For this review, take the finished solid that the model builds, in its own axes (mm). A direction names the side the tool comes from. Coordinates: 2 decimals unless noted, no trailing zeros. Write each loop counter-clockwise with the first axis right and the second up, starting at its lowest first coordinate (ties: lowest second). Pieces come first, ordered by that corner, then holes. Notation, with made-up numbers: (31, -36.75) -> (88, -36.75) arc R23 ccw to (88, -20.75) -> close; hole circle Ø7 at (6.25, -36). An arc over 180 degrees is marked (long way). One line per item, written item: value. Start each with the question number.
1) Add section A-A (z = -6.5). State the section outline as (x, y) points, and give its area (3 significant figures).
2) For probe 1 along X at (y, z) = (13, -11.5); probe 2 along Z at (x, y) = (27.5, -68.5); probe 3 along Y at (x, z) = (-10, -6.5), list the stretches that pass through material, from the lowest coordinate up. Write a range as from..to.
3) Machinability: for faces 4 (the flat face through (11, 70, -7)), 5 (the flat face through (11, -70, -7)), 6 (the flat face through (-7, -1, -7)), 7 (the flat face through (-15, -1, -7)), 8 (the flat face through (15, -1, -7)), which of the approach directions +Z, -Z, +X, -X, +Y, -Y give a long, thin tool a straight path to every point of the face, cutting with its end or side? Answer none if there is none.
4) Mouldability with a two-part tool opening along X and no side actions: class faces 1 (the flat face through (7, -1, -7)), 2 (the flat face through (-1, -90, 2)), 3 (the flat face through (-60, -3, 2)) as released by +X, released by -X, zero draft, split by the parting line, or undercut.
5) Add section B-B (y = -6.5). State the section outline as (x, z) points, and give its area (3 significant figures).
6) For pin 1 Ø8 at (x, y) = (22, 8.5) entering from -Z; pin 2 Ø1.5 at (y, z) = (-28.5, -11) entering from +X; pin 3 Ø4 at (x, z) = (-12.5, -9) entering from +Y, all flat-tipped, find the tip position at first contact; note any pin that passes through.
7) Add section C-C (x = -1.5). State the section outline as (y, z) points, and give its area (4 significant figures).
8) Add section D-D (y = -76). State the section outline as (x, z) points, and give its area (3 significant figures).
from build123d import *

# Parameters (mm, degrees)
SKETCH1_W           = 120
SKETCH1_H           = 180
BOSS_EXTRUDE1_DEPTH = 5
SKETCH2_W           = 8
SKETCH2_H           = 140
BOSS_EXTRUDE2_DEPTH = 14
SKETCH3_W           = 120
SKETCH3_H           = 3.5
CUT_EXTRUDE1_DEPTH  = 10


with BuildPart() as part:
    # Sketch1 → Boss-Extrude1 (new body)
    with BuildSketch(Plane.XY):
        Rectangle(SKETCH1_W, SKETCH1_H)
    extrude(amount=BOSS_EXTRUDE1_DEPTH)

    # Sketch2 → Boss-Extrude2 (add)
    with BuildSketch(Plane(origin=(0, 0, 0), x_dir=(-1, 0, 0), z_dir=(0, 0, -1))):
        with Locations((-11, 0)):
            Rectangle(SKETCH2_W, SKETCH2_H)
        with Locations((11, 0)):
            Rectangle(SKETCH2_W, SKETCH2_H)
    extrude(amount=BOSS_EXTRUDE2_DEPTH)

    # Sketch3 → Cut-Extrude1 (cut)
    with BuildSketch(Plane(origin=(0, 0, 0), x_dir=(-1, 0, 0), z_dir=(0, 0, -1))):
        with Locations((0, 88.25)):
            Rectangle(SKETCH3_W, SKETCH3_H)
    extrude(amount=-CUT_EXTRUDE1_DEPTH, mode=Mode.SUBTRACT)


solid = part.part
Numbers:
1. outline: (-15, -70) -> (-7, -70) -> (-7, 70) -> (-15, 70) -> close; (7, -70) -> (15, -70) -> (15, 70) -> (7, 70) -> close
1. area: 2,240 mm²
2. probe 1: -15..-7, 7..15
2. probe 2: 0..5
2. probe 3: -70..70
3. face 4: -Z, +X, -X, +Y
3. face 5: -Z, +X, -X, -Y
3. face 6: -Z, +Y, -Y
3. face 7: -Z, -X, +Y, -Y
3. face 8: -Z, +X, +Y, -Y
4. face 1: undercut
4. face 2: zero draft
4. face 3: released by -X
5. outline: (-60, 0) -> (-15, 0) -> (-15, -14) -> (-7, -14) -> (-7, 0) -> (7, 0) -> (7, -14) -> (15, -14) -> (15, 0) -> (60, 0) -> (60, 5) -> (-60, 5) -> close
5. area: 824 mm²
6. pin 1: z = 0
6. pin 2: x = 15
6. pin 3: y = 70
7. outline: (-90, 0) -> (86.5, 0) -> (86.5, 5) -> (-90, 5) -> close
7. area: 882.5 mm²
8. outline: (-60, 0) -> (60, 0) -> (60, 5) -> (-60, 5) -> close
8. area: 600 mm²
